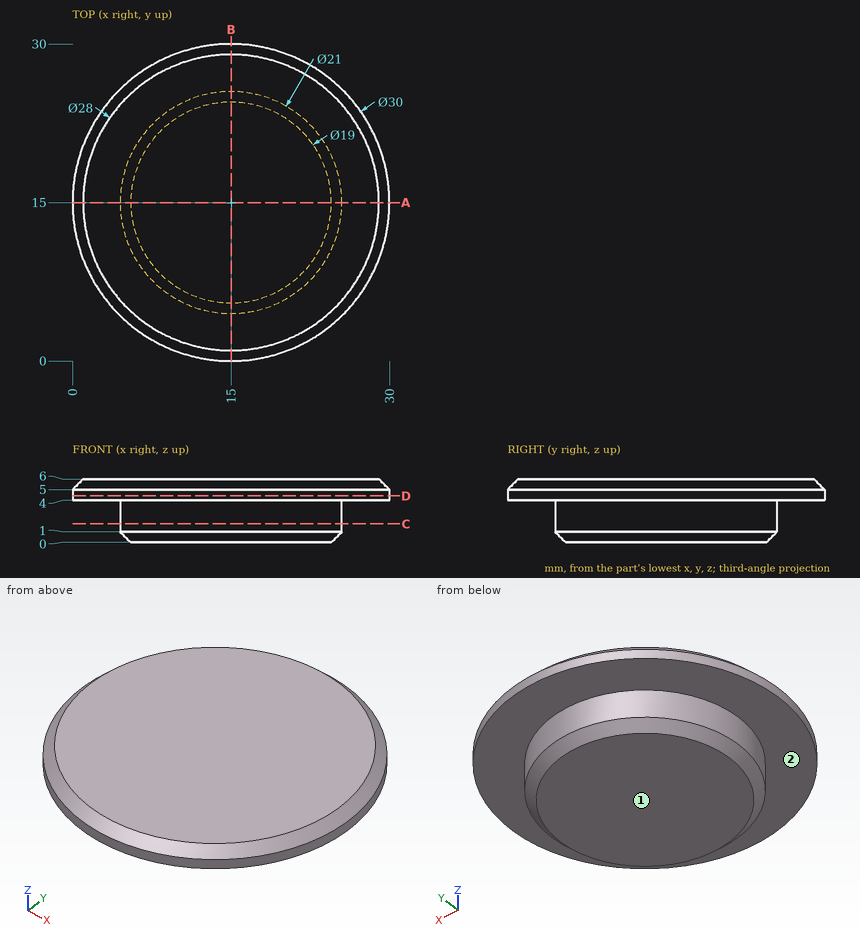
Could you check a few things on this drawing? It's one solid part, dimensions in mm from its lowest x, y, z. A direction names the side the tool comes from. Coordinates: 2 decimals unless noted, no trailing zeros. Write each loop counter-clockwise with the first axis right and the second up, starting at its lowest first coordinate (ties: lowest second). Pieces come first, ordered by that corner, then holes.
Q1. Imagine slicing it at C-C, the plane z = 1.75. List the corners of the cut face in (x, y) for me, plus the area to 3 significant figures.
Results found:
outline: circle Ø21 at (15, 15)
area: 346 mm2
Q2. Imagine slicing it at D-D, the plane z = 4.4. List the corners of the cut face in (x, y) for me, plus the area to 3 significant figures.
Results found:
outline: circle Ø30 at (15, 15)
area: 707 mm2
Q3. For P1, Ø3, axis at x = 17.5, z = 4, coming from the +Y side, with a flat end and sliding along its axis, tell me the tip position at first contact or that it passes through.
Results found:
P1: stops at y = 29.97
Q4. Which directions (+Z, -Z, +X, -X, +Y, -Y) give clear straight access to the entire face, cutting with the end or side of a thin tool? Please do the marked faces 1 and 2.
Results found:
face 1: -Z, +X, -X, +Y, -Y
face 2: -Z
Q5. Imagine slicing it at A-A, the plane y = 15. List the corners of the cut face in (x, z) for me, plus the area to 3 significant figures.
Results found:
outline: (0, 4) - (4.5, 4) - (4.5, 1) - (5.5, 0) - (24.5, 0) - (25.5, 1) - (25.5, 4) - (30, 4) - (30, 5) - (29, 6) - (1, 6) - (0, 5) - close
area: 142 mm2
Q6. Please list where these lines run through material, in increasing order: L1, parallel to Z at x = 22.5, y = 25.5; L2, parallel to X at y = 5.5, z = 1.65; L3, parallel to Y at x = 14.75, z = 4.7.
Results found:
L1: z = 4 to 6
L2: x = 10.53 to 19.47
L3: y = 0 to 30
